from build123d import *

# Parameters (mm, degrees)
F1_DEPTH = 74.676
F2_W     = 65.046132
F2_H     = 38.793292
F3_DEPTH = 123.19
F4_W     = 75.36434
F4_H     = 42.812191
F5_DEPTH = 78.74
F6_W     = 15.368398
F6_H     = 37.422214
F7_DEPTH = 116.84


with BuildPart() as f1:
    # F0 (on Top) → F1 (new body)
    with BuildSketch(Plane.XY):
        Polygon((-37.479065, 17.799251), (-62.800989, 17.799251), (-62.800989, -30.872758), (69.400154, -30.872758), (-37.479065, 0), align=None)
    extrude(amount=F1_DEPTH)

    # F2 (on Top) → F3 (cut)
    with BuildSketch(Plane.XY):
        with Locations((-32.523066, 19.396646)):
            Rectangle(F2_W, F2_H)
    extrude(amount=F3_DEPTH, mode=Mode.SUBTRACT)

    # F4 (on Top) → F5 (cut)
    with BuildSketch(Plane.XY):
        with Locations((-96.438488, -21.406095)):
            Rectangle(F4_W, F4_H)
    extrude(amount=F5_DEPTH, mode=Mode.SUBTRACT)

    # F6 (on Top) → F7 (cut)
    with BuildSketch(Plane.XY):
        with Locations((-58.310846, -18.711107)):
            Rectangle(F6_W, F6_H)
    extrude(amount=F7_DEPTH, mode=Mode.SUBTRACT)


solid = f1.part
Design review of the part built by this model. Coordinates are the model's own, in mm. Give positions to 0.01 mm unless a question says otherwise; leave off trailing zeros. Loops run counter-clockwise (first coordinate to the right, second up) from the corner with the lowest first, then second, coordinate; pieces in that order, holes last. Notation, with made-up numbers: M 36.5,-2.75 L 42.5,-2.75 A15 cw 42.5,18.25 Z; hole C -10.75,33.5 d4. An arc over 180 degrees is marked long. Answer as a JSON object with one key per item and string values.
Item 1: We need section B-B (y = -10). State the section outline as (x, z) points, and give its area (3 significant figures).
Output values:
{"outline": "M -50.63,0 L -2.86,0 L -2.86,74.68 L -50.63,74.68 Z", "area": "3,570 mm2"}
Item 2: We need section A-A (z = 43). State the section outline as (x, y) points, and give its area (3 significant figures).
Output values:
{"outline": "M -50.63,-30.87 L 69.4,-30.87 L -37.48,0 L -50.63,0 Z", "area": "2,060 mm2"}
Item 3: Wall thickness on line 1 along Y through (x, z) = (-1, 47.5); line 2 along Y through (x, z) = (9, 11.5): over which ranges is each line inside the solid? List them lowest first.
Output values:
{"line 1": "y = -30.87 to -10.54", "line 2": "y = -30.87 to -13.43"}
Item 4: For P1, Ø1.5, axis at x = 33, z = 14.5, coming from the +Y side, flat-tipped, find the tip position at first contact; note if it passes through.
Output values:
{"P1": "stops at y = -20.14"}
